Geometry: final body of the model. Coordinates: model frame, mm. Face numbers are marked on the shaded views. A direction names the side the tool comes from. Give positions to 0.01 mm unless a question says otherwise; leave off trailing zeros. Write each loop counter-clockwise with the first axis right and the second up, starting at its lowest first coordinate (ties: lowest second). Pieces come first, ordered by that corner, then holes. Notation, with made-up numbers: (25.5, 74) -> (58.5, 74) arc R20 ccw to (58.5, 113) -> close; hole circle Ø11 at (8, -12). An arc over 180 degrees is marked (long way). Use CSV: the item, a comma, the result in double quotes. Start each with the question number.
1) Section C-C (x = 0). Output: boundary loops of the cut face in (y, z), plus the area to 3 significant figures.
2) Set-up query: the marked faces 1 and 2. Return all of +Z, -Z, +X, -X, +Y, -Y with unobstructed straight access to the full face (end or side cutting, diameter ignored); none if empty.
3) Section B-B (y = -43). Output: boundary loops of the cut face in (x, z).
4) Material intervals for line 1 (Z direction, x = -7, y = -5.5); line 2 (Z direction, x = 18, y = 2); line 3 (X direction, y = -21, z = -8), sorted ascending. Write a range as [from, to].
5) Section D-D (y = -27). Output: boundary loops of the cut face in (x, z), plus the area to 3 significant figures.
6) Section A-A (z = 0). Output: boundary loops of the cut face in (x, y), plus the area to 3 significant figures.
7) Contact query for flat-ended pins moving along their axis: P1, Ø3, axis at x = 6.5, y = 7.5, coming from the +Z side; P2, Ø6, axis at x = 2, z = 3.5, coming from the +Y side; P3, Ø3, axis at x = -3.5, y = 8, coming from the +Z side. Output: stop coordinate, or through.
```python
from build123d import *

# Parameters (mm, degrees)
CUT_EXTRUDE1_DEPTH      = 52.961524227
CUT_EXTRUDE1_DEPTH_BACK = 52.961524227
SHELL1_T                = -1


with BuildPart() as part:
    # Sketch1 → Revolve1 (revolve)
    with BuildSketch(Plane.XY):
        with BuildLine():
            Line((0, 30), (0, -30))
            ThreePointArc((0, -30), (30, 0), (0, 30))
        make_face()
    revolve(axis=Axis((0, 30, 0), (0, -1, 0)))

    # Sketch2 → Cut-Extrude1 (cut, two sides: drawn at the far end of the back side and taken through both)
    with BuildSketch(Plane.XY.offset(-CUT_EXTRUDE1_DEPTH_BACK)):
        Polygon((-219.842197388, 15), (-39.041394336, 15), (42.58256389, 15), (223.383366942, 15), (223.383366942, 376.601606104), (-219.842197388, 376.601606104), align=None)
    extrude(amount=CUT_EXTRUDE1_DEPTH + CUT_EXTRUDE1_DEPTH_BACK, mode=Mode.SUBTRACT)

    # Shell1
    shell1_openings = [part.faces().sort_by_distance(p)[0] for p in [
        (0, 15, 0),
    ]]
    offset(amount=SHELL1_T, openings=shell1_openings, kind=Kind.INTERSECTION)

    # Sketch3 → Revolve2 (revolve)
    with BuildSketch(Plane.XY):
        with BuildLine():
            Line((0, -30), (0, -55))
            Line((0, -55), (10, -55))
            Line((10, -55), (10, -28.284271247))
            ThreePointArc((10, -28.284271247), (5.073059362, -29.56795679), (0, -30))
        make_face()
    revolve(axis=Axis((0, -30, 0), (0, -1, 0)))


solid = part.part
```
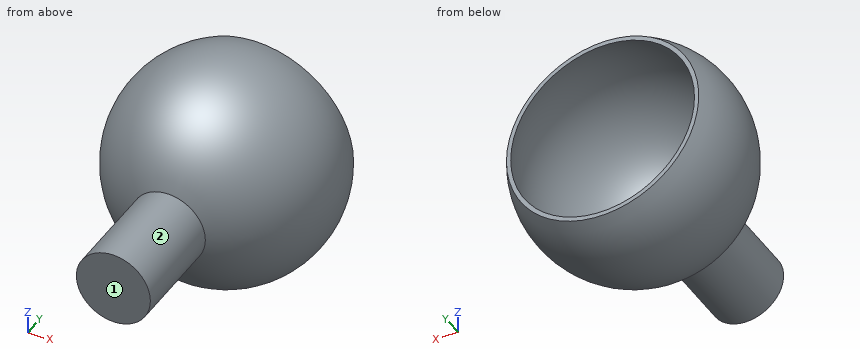
Answers follow:
1,outline,"(-55, -10) -> (-28.28, -10) arc R30 ccw to (15, -25.98) -> (15, -24.82) arc R29 cw (long way) to (15, 24.82) -> (15, 25.98) arc R30 ccw to (-28.28, 10) -> (-55, 10) -> close"
1,area,"635 mm^2"
2,face 1,"+Z, -Z, +X, -X, -Y"
2,face 2,"-Y"
3,outline,"circle Ø20 at (0, 0)"
4,line 1,"z = [-28.65, -27.6], [27.6, 28.65]"
4,line 2,"z = [-23.92, -22.65], [22.65, 23.92]"
4,line 3,"x = [-19.87, -18.33], [18.33, 19.87]"
5,outline,"circle Ø26.15 at (0, 0); hole circle Ø21.17 at (0, 0)"
5,area,"185 mm^2"
6,outline,"(-25.98, 15) arc R30 ccw to (-10, -28.28) -> (-10, -55) -> (10, -55) -> (10, -28.28) arc R30 ccw to (25.98, 15) -> (24.82, 15) arc R29 cw (long way) to (-24.82, 15) -> close"
6,area,"635 mm^2"
7,P1,"stops at z = 28.79"
7,P2,"stops at y = -28.13"
7,P3,"stops at z = 29.12"
